Geometry: see drawing. Coordinates: mm, zero at the bounding-box minimum. A direction names the side the tool comes from. Give positions to 0.01 mm unless a question says otherwise; leave off trailing zeros. Order: outer loops, then holes, each group sorted by start corner. A loop starts at its lowest first (then second) coordinate and runs counter-clockwise, first axis right, second up. Notation, with made-up numbers: (-18, -17.5) - (12, -17.5) arc R35 cw to (12, 16.5) - close; hole circle Ø1 at (75, 9.5). An arc over 180 degrees is marked (long way). Put each result on its own line as item: value. Start each with the question number.
1. Mould query, pull axis X, two halves, no side actions, for the marked faces 1, 2 and 3. Classes: pulls with the +X half, pulls with the -X half, needs draft (parallel to the pull), parting line crosses it, or undercut.
2. First-contact query: P1, Ø3, axis at y = 55, z = 2, coming from the -X side; P2, Ø11, axis at x = 28, z = 16.5, coming from the +Y side; P3, Ø12, axis at x = 9, y = 50, coming from the +Z side; P4, Ø3, axis at x = 28, y = 51, coming from the +Z side. Flat tips, straight axial feed; report the tip coordinate or a pass-through.
3. Section D-D on y = 51. Return the cut outline in (x, z).
4. Section C-C on z = 31. Return the cut outline in (x, y).
5. Section A-A on x = 28. Return the cut outline in (y, z).
6. Section B-B on z = 3. Return the cut outline in (x, y).
7. Ray query, line 1 along X through (y, z) = (3, 31); line 2 along Z through (x, y) = (34.9, 0.95); line 3 along Z through (x, y) = (38.5, 53.5). Return the intervals inside material, ascending. Write a range as from..to.
8. Set-up query: the marked faces 4 and 5. Return all of +Z, -Z, +X, -X, +Y, -Y with unobstructed straight access to the full face (end or side cutting, diameter ignored); none if empty.
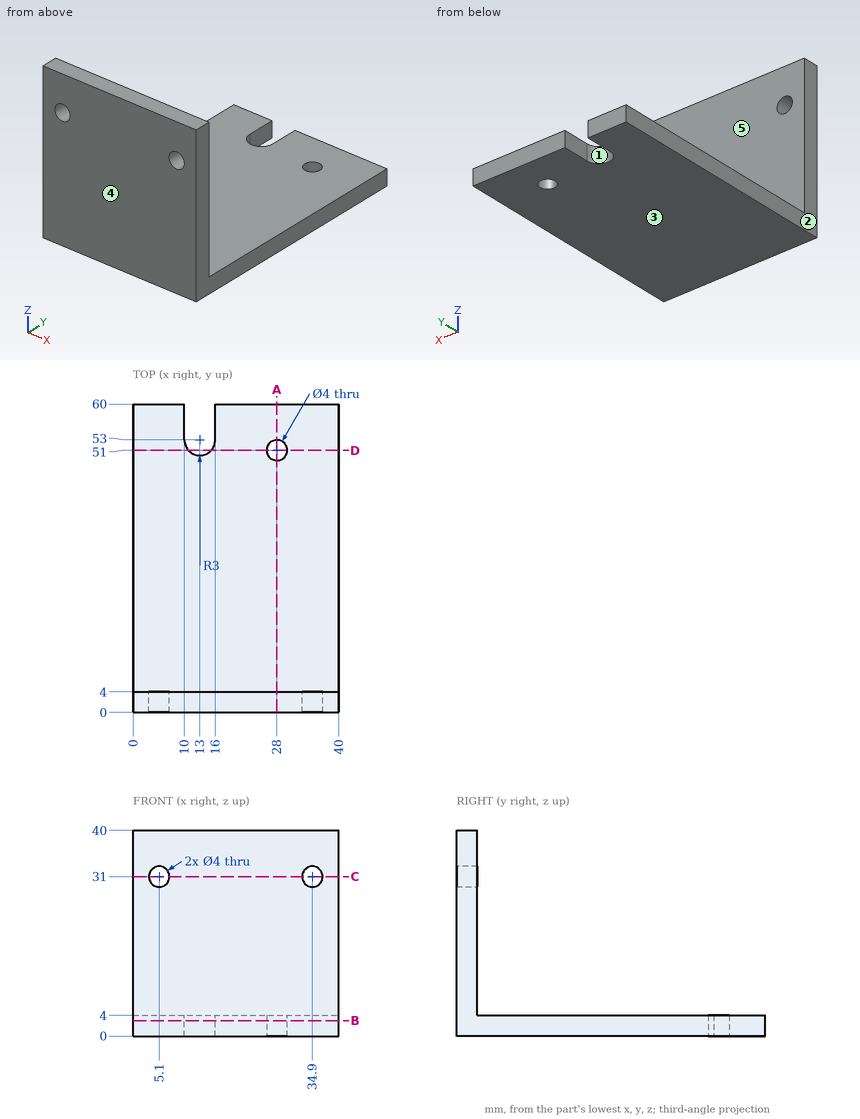
Resolved:
1. face 1: undercut
1. face 2: pulls with the -X half
1. face 3: needs draft
2. P1: x = 0
2. P2: y = 4
2. P3: z = 4
2. P4: through
3. outline: (0, 0) - (10.76, 0) - (10.76, 4) - (0, 4) - close; (15.24, 0) - (26, 0) - (26, 4) - (15.24, 4) - close; (30, 0) - (40, 0) - (40, 4) - (30, 4) - close
4. outline: (0, 0) - (3.1, 0) - (3.1, 4) - (0, 4) - close; (7.1, 0) - (32.9, 0) - (32.9, 4) - (7.1, 4) - close; (36.9, 0) - (40, 0) - (40, 4) - (36.9, 4) - close
5. outline: (0, 0) - (49, 0) - (49, 4) - (4, 4) - (4, 40) - (0, 40) - close; (53, 0) - (60, 0) - (60, 4) - (53, 4) - close
6. outline: (0, 0) - (40, 0) - (40, 60) - (16, 60) - (16, 53) arc R3 cw to (10, 53) - (10, 60) - (0, 60) - close; hole circle Ø4 at (28, 51)
7. line 1: 0..3.1, 7.1..32.9, 36.9..40
7. line 2: 0..29, 33..40
7. line 3: 0..4
8. face 4: +Z, -Z, +X, -X, -Y
8. face 5: +Z, +X, -X, +Y
